Here's how the part is built. I have some questions about the finished solid (model axes, mm). Face numbers are marked on the shaded views. A direction names the side the tool comes from. Coordinates: 2 decimals unless noted, no trailing zeros. Write each loop counter-clockwise with the first axis right and the second up, starting at its lowest first coordinate (ties: lowest second). Pieces come first, ordered by that corner, then holes.
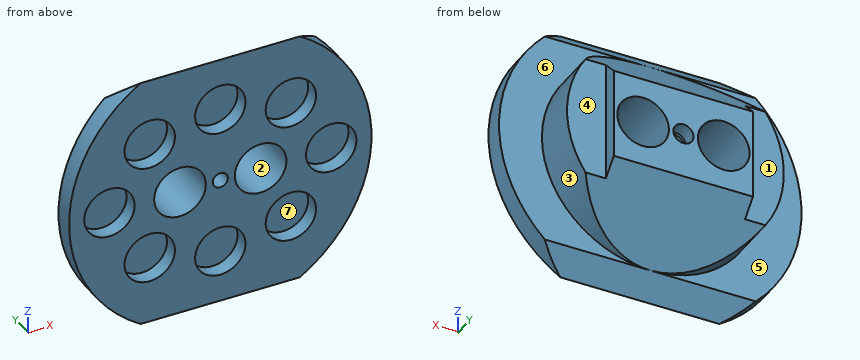
from build123d import *
from build123d.topology import SkipClean

# Parameters (mm, degrees)
SKETCH1_R                            = 30
BOSS_EXTRUDE1_DEPTH                  = 4
BOSS_EXTRUDE2_REACH                  = 44.615
BOSS_EXTRUDE2_END_RADIUS             = 30
BOSS_EXTRUDE2_DIRECTION_2_REACH      = 44.615
BOSS_EXTRUDE2_DIRECTION_2_END_RADIUS = 30
SKETCH3_OUTSIDE_W                    = 78.092
SKETCH3_OUTSIDE_H                    = 69.092
SKETCH3_OUTSIDE_R                    = 21.5
CUT_EXTRUDE2_DEPTH                   = 12.5
BOSS_EXTRUDE3_DEPTH                  = 18
BOSS_EXTRUDE4_DEPTH                  = 15
BOSS_EXTRUDE5_DEPTH                  = 15
CUT_EXTRUDE3_DEPTH                   = 44.292609069
CUT_EXTRUDE3_DEPTH_BACK              = 44.292609069
SKETCH8_R                            = 2
CUT_EXTRUDE8_DEPTH                   = 48.077064479
CUT_EXTRUDE8_DEPTH_BACK              = 48.077064479
CUT_EXTRUDE9_DEPTH                   = 59.659818207
CUT_EXTRUDE11_DEPTH                  = 20
CUT_EXTRUDE12_DEPTH                  = 20
CUT_EXTRUDE13_DEPTH                  = 20
CUT_EXTRUDE14_DEPTH                  = 44.292609069
CUT_EXTRUDE14_DEPTH_BACK             = 44.292609069
SKETCH25_W                           = 66.075437062
SKETCH25_H                           = 20.142243048
SKETCH26_R                           = 5.125
CUT_EXTRUDE15_DEPTH                  = 24
CUT_EXTRUDE17_DEPTH                  = 47.524187258
CUT_EXTRUDE17_DEPTH_BACK             = 47.524187258
SKETCH29_W                           = 7.7
SKETCH29_H                           = 3
CUT_EXTRUDE18_DEPTH                  = 47.524187258
CUT_EXTRUDE18_DEPTH_BACK             = 47.524187258
SKETCH31_W                           = 7.7
SKETCH31_H                           = 3
SKETCH34_R                           = 1.5
CUT_EXTRUDE21_DEPTH                  = 20
SKETCH35_R                           = 2
CUT_EXTRUDE22_DEPTH                  = 3
SKETCH37_R                           = 5
CUT_EXTRUDE23_DEPTH                  = 3


with BuildPart() as part:
    # Sketch1 → Boss-Extrude1 (new body)
    with BuildSketch(Plane(origin=(0, 0, 0), x_dir=(1, 0, 0), z_dir=(0, 1, 0))):
        with Locations(Location((0, 0, 0), (0, 0, 270))):
            Circle(SKETCH1_R)
    extrude(amount=BOSS_EXTRUDE1_DEPTH)

    # Boss-Extrude2: up to this cylinder (the profile starts inside it)
    with SkipClean():  # the faces are left unmerged after this step: merging them gives an invalid solid
        boss_extrude2_end = Plane(origin=(0, 9.396175, 0), z_dir=(0, -1, 0)) * Cylinder(BOSS_EXTRUDE2_END_RADIUS, 150.23, mode=Mode.PRIVATE)
        # Sketch2 → Boss-Extrude2 (add, up to the surface)
        with BuildSketch(Plane(origin=(0, 0, 0), x_dir=(0, 0, -1), z_dir=(1, 0, 0)), mode=Mode.PRIVATE) as boss_extrude2_sk1:
            Polygon((0, 4), (21.5, 4), (9, 16.5), (-9, 16.5), (-21.5, 4), align=None)
        boss_extrude2_tool1 = extrude(boss_extrude2_sk1.sketch, amount=BOSS_EXTRUDE2_REACH, mode=Mode.PRIVATE) & boss_extrude2_end
        add(boss_extrude2_tool1.solids().sort_by_distance((0, 9.396175, 0))[0])

    # Boss-Extrude2 direction 2: up to this cylinder (the profile starts inside it)
    with SkipClean():  # the faces are left unmerged after this step: merging them gives an invalid solid
        boss_extrude2_direction_2_end = Plane(origin=(0, 9.396175, 0), z_dir=(0, -1, 0)) * Cylinder(BOSS_EXTRUDE2_DIRECTION_2_END_RADIUS, 150.23, mode=Mode.PRIVATE)
        # Sketch2 → Boss-Extrude2 direction 2 (add, up to the surface)
        with BuildSketch(Plane(origin=(0, 0, 0), x_dir=(0, 0, -1), z_dir=(1, 0, 0)), mode=Mode.PRIVATE) as boss_extrude2_direction_2_sk1:
            Polygon((0, 4), (21.5, 4), (9, 16.5), (-9, 16.5), (-21.5, 4), align=None)
        boss_extrude2_direction_2_tool1 = extrude(boss_extrude2_direction_2_sk1.sketch, amount=-BOSS_EXTRUDE2_DIRECTION_2_REACH, mode=Mode.PRIVATE) & boss_extrude2_direction_2_end
        add(boss_extrude2_direction_2_tool1.solids().sort_by_distance((0, 9.396175, 0))[0])

    # SurfaceCut1
    split(bisect_by=Plane(origin=(0, 12.75, -12.75), x_dir=(1, 0, 0), z_dir=(0, 0.7071067811865558, -0.7071067811865392)), keep=Keep.BOTTOM)

    # SurfaceCut2
    split(bisect_by=Plane(origin=(0, 12.75, 12.75), x_dir=(1, 0, 0), z_dir=(0, 0.7071067811865509, 0.7071067811865442)), keep=Keep.BOTTOM)

    # Sketch3 outside → Cut-Extrude2 (cut)
    with BuildSketch(Plane(origin=(0, 4, 0), x_dir=(1, 0, 0), z_dir=(0, 1, 0))):
        Rectangle(SKETCH3_OUTSIDE_W, SKETCH3_OUTSIDE_H)
        Circle(SKETCH3_OUTSIDE_R, mode=Mode.SUBTRACT)
    extrude(amount=CUT_EXTRUDE2_DEPTH, mode=Mode.SUBTRACT)

    # Sketch5 → Boss-Extrude3 (add)
    with BuildSketch(Plane(origin=(0, 0, 0), x_dir=(-1, 0, 0), z_dir=(0, -1, 0))):
        Polygon((0, -6), (-17.5, -6), (-17.5, 6), (17.5, 6), (17.5, -6), align=None)
    extrude(amount=BOSS_EXTRUDE3_DEPTH)

    # Sketch6 → Boss-Extrude4 (add)
    with BuildSketch(Plane.XZ):
        Polygon((0, 15), (7, 15), (7, 6), (-7, 6), (-7, 15), align=None)
    extrude(amount=BOSS_EXTRUDE4_DEPTH)

    # Sketch7 → Boss-Extrude5 (add)
    with BuildSketch(Plane.XZ):
        Polygon((0, -15), (7, -15), (7, -6), (-7, -6), (-7, -15), align=None)
    extrude(amount=BOSS_EXTRUDE5_DEPTH)

    # Sketch8 → Cut-Extrude3 (cut, two sides: drawn at the far end of the back side and taken through both)
    with BuildSketch(Plane.XY.offset(-CUT_EXTRUDE3_DEPTH_BACK)):
        with Locations((-12.5, -12.5)):
            Circle(SKETCH8_R)
        with Locations((12.5, -12.5)):
            Circle(SKETCH8_R)
    extrude(amount=CUT_EXTRUDE3_DEPTH + CUT_EXTRUDE3_DEPTH_BACK, mode=Mode.SUBTRACT)

    # Sketch16 → Cut-Extrude8 (cut, two sides: drawn at the far end of the back side and taken through both)
    with BuildSketch(Plane.XY.offset(6).offset(-CUT_EXTRUDE8_DEPTH_BACK)):
        Polygon((17.5, -18), (17.5, -14.5), (14, -18), align=None)
        Polygon((-17.5, -18), (-14, -18), (-17.5, -14.5), align=None)
    extrude(amount=CUT_EXTRUDE8_DEPTH + CUT_EXTRUDE8_DEPTH_BACK, mode=Mode.SUBTRACT)

    # Sketch17 → Cut-Extrude9 (cut, through all)
    with BuildSketch(Plane(origin=(10.365975269, -9.674910251, -8.062425209), x_dir=(-0.3613483622370374, 0.337258471421235, -0.8693009171531012), z_dir=(0.6355070151731325, -0.5931398808282571, -0.49428323402354774))):
        Polygon((-2.372510104, -6.189601271), (7.980636686, -0.706686759), (7.980636686, -10.965829024), align=None)
    extrude(amount=CUT_EXTRUDE9_DEPTH, mode=Mode.SUBTRACT)

    # Sketch19 → Cut-Extrude11 (cut)
    with BuildSketch(Plane(origin=(-10.365975269, -9.674910251, -8.062425209), x_dir=(0.3613483622370374, 0.33725847142123494, -0.8693009171531012), z_dir=(0.6355070151731324, 0.5931398808282571, 0.4942832340235476))):
        Polygon((-2.372510104, -6.189601271), (7.980636686, -10.965829024), (7.980636686, -0.706686759), align=None)
    extrude(amount=-CUT_EXTRUDE11_DEPTH, mode=Mode.SUBTRACT)

    # Sketch20 → Cut-Extrude12 (cut)
    with BuildSketch(Plane(origin=(-10.365975269, -9.674910251, 8.062425209), x_dir=(-0.3613483622370374, -0.3372584714212349, -0.8693009171531013), z_dir=(0.6355070151731326, 0.593139880828257, -0.49428323402354757))):
        Polygon((2.372510104, -6.189601271), (-7.980636686, -0.706686759), (-7.980636686, -10.965829024), align=None)
    extrude(amount=-CUT_EXTRUDE12_DEPTH, mode=Mode.SUBTRACT)

    # Sketch21 → Cut-Extrude13 (cut)
    with BuildSketch(Plane(origin=(10.365975269, -9.674910251, 8.062425209), x_dir=(-0.3613483622370374, 0.3372584714212349, 0.8693009171531013), z_dir=(-0.6355070151731326, 0.593139880828257, -0.49428323402354757))):
        Polygon((-2.372510104, -6.189601271), (7.980636686, -0.706686759), (7.980636686, -10.965829024), align=None)
    extrude(amount=-CUT_EXTRUDE13_DEPTH, mode=Mode.SUBTRACT)

    # Sketch25 → Cut-Extrude14 (cut, two sides: drawn at the far end of the back side and taken through both)
    with BuildSketch(Plane.XY.offset(-CUT_EXTRUDE14_DEPTH_BACK)):
        with Locations((0, -10.071121524)):
            Rectangle(SKETCH25_W, SKETCH25_H)
    extrude(amount=CUT_EXTRUDE14_DEPTH + CUT_EXTRUDE14_DEPTH_BACK, mode=Mode.SUBTRACT)

    # Sketch26 → Cut-Extrude15 (cut)
    with BuildSketch(Plane(origin=(0, 16.5, 0), x_dir=(1, 0, 0), z_dir=(0, 1, 0))):
        with Locations(Location((-8, 0, 0), (0, 0, 270))):
            Circle(SKETCH26_R)
        with Locations(Location((8, 0, 0), (0, 0, 270))):
            Circle(SKETCH26_R)
    extrude(amount=-CUT_EXTRUDE15_DEPTH, mode=Mode.SUBTRACT)

    # Sketch29 → Cut-Extrude17 (cut, two sides: drawn at the far end of the back side and taken through both)
    with BuildSketch(Plane.XY.offset(6).offset(-CUT_EXTRUDE17_DEPTH_BACK)):
        with Locations((17.65, 15)):
            Rectangle(SKETCH29_W, SKETCH29_H)
    extrude(amount=CUT_EXTRUDE17_DEPTH + CUT_EXTRUDE17_DEPTH_BACK, mode=Mode.SUBTRACT)

    # Sketch31 → Cut-Extrude18 (cut, two sides: drawn at the far end of the back side and taken through both)
    with BuildSketch(Plane.XY.offset(6).offset(-CUT_EXTRUDE18_DEPTH_BACK)):
        with Locations((-17.65, 15)):
            Rectangle(SKETCH31_W, SKETCH31_H)
    extrude(amount=CUT_EXTRUDE18_DEPTH + CUT_EXTRUDE18_DEPTH_BACK, mode=Mode.SUBTRACT)

    # Sketch34 → Cut-Extrude21 (cut)
    with BuildSketch(Plane.XZ):
        with Locations(Location((0, 0, 0), (0, 0, 270))):
            Circle(SKETCH34_R)
    extrude(amount=-CUT_EXTRUDE21_DEPTH, mode=Mode.SUBTRACT)

    # Sketch35 → Cut-Extrude22 (cut)
    with BuildSketch(Plane(origin=(0, 16.5, 0), x_dir=(1, 0, 0), z_dir=(0, 1, 0))):
        with Locations(Location((0, 0, 0), (0, 0, 270))):
            Circle(SKETCH35_R)
    extrude(amount=-CUT_EXTRUDE22_DEPTH, mode=Mode.SUBTRACT)

    # Sketch37 → Cut-Extrude23 (cut)
    with BuildSketch(Plane.XZ):
        with Locations(Location((0, -15, 0), (0, 0, 270))):
            Circle(SKETCH37_R)
        with Locations(Location((0, 15, 0), (0, 0, 270))):
            Circle(SKETCH37_R)
        with Locations(Location((-22, 0, 0), (0, 0, 270))):
            Circle(SKETCH37_R)
        with Locations(Location((22, 0, 0), (0, 0, 270))):
            Circle(SKETCH37_R)
        with Locations(Location((-14, 12, 0), (0, 0, 270))):
            Circle(SKETCH37_R)
        with Locations(Location((14, 12, 0), (0, 0, 270))):
            Circle(SKETCH37_R)
        with Locations(Location((-14, -12, 0), (0, 0, 270))):
            Circle(SKETCH37_R)
        with Locations(Location((14, -12, 0), (0, 0, 270))):
            Circle(SKETCH37_R)
    extrude(amount=-CUT_EXTRUDE23_DEPTH, mode=Mode.SUBTRACT)


solid = part.part
1. Thinking about a two-plate mould opening in Z: for the marked faces 1, 2 and 3, which applies, pulls with the +Z half, pulls with the -Z half, needs draft (parallel to the pull), parting line crosses it, or undercut?
2. I want a section at B-B (x = 12). List the corners of the cut face in (y, z) for me.
3. I want a section at C-C (z = -3.5). List the corners of the cut face in (x, y) for me, then the cut area to 3 significant figures.
4. I want a section at D-D (z = -13.5). List the corners of the cut face in (x, y) for me.
5. If I drill on line 1 (X direction, y = 1.2, z = 0) (3 decimals); line 2 (X direction, y = 9.25, z = 0) (3 decimals); line 3 (X direction, y = 12.75, z = -4), over which ranges is the centre line in solid material (lowest first)?
6. On a 3-axis mill with a long thin cutter (end or side, diameter ignored), from which of +Z, -Z, +X, -X, +Y, -Y can I reach the whole of each face in a straight line? I mean the marked faces 4, 5, 6 and 7. Say none if no direction works.
7. I want a section at A-A (y = 14.75). List the corners of the cut face in (x, z) for me (3 decimals).
8. For pin 1 Ø5 at (x, z) = (21.5, 2) entering from -Y; pin 2 Ø16 at (x, z) = (0, 15) entering from -Y; pin 3 Ø1.5 at (y, z) = (15.5, 5.5) entering from +X; pin 4 Ø9 at (x, z) = (-20, 3) entering from +Y, each with a flat end and sliding along its axis, tell me the tip position at first contact or that it passes through.
Response values:
1. face 1: needs draft
1. face 2: undercut
1. face 3: parting line crosses it
2. outline: (0, -25.5) - (4, -21.5) - (4, -17.84) - (7.66, -17.84) - (16.5, -9) - (16.5, -3.2) - (0, -3.2) - (0, -7.42) - (3, -7.42) - (3, -16.58) - (0, -16.58) - close; (0, 3.2) - (16.5, 3.2) - (16.5, 9) - (7.66, 17.84) - (4, 17.84) - (4, 21.5) - (0, 25.5) - (0, 16.58) - (3, 16.58) - (3, 7.42) - (0, 7.42) - close
3. outline: (-29.8, 0) - (-25.57, 0) - (-25.57, 3) - (-18.43, 3) - (-18.43, 0) - (-11.74, 0) - (-11.74, 16.5) - (-13.8, 16.5) - (-13.8, 13.5) - (-21.21, 13.5) - (-21.21, 4) - (-29.8, 4) - close; (-4.26, 0) - (4.26, 0) - (4.26, 16.5) - (-4.26, 16.5) - close; (11.74, 0) - (18.43, 0) - (18.43, 3) - (25.57, 3) - (25.57, 0) - (29.8, 0) - (29.8, 4) - (21.21, 4) - (21.21, 13.5) - (13.8, 13.5) - (13.8, 16.5) - (11.74, 16.5) - close
3. area: 434 mm2
4. outline: (-26.79, 0) - (-18.77, 0) - (-18.77, 3) - (-9.23, 3) - (-9.23, 0) - (-4.77, 0) - (-4.77, 3) - (4.77, 3) - (4.77, 0) - (9.23, 0) - (9.23, 3) - (18.77, 3) - (18.77, 0) - (26.79, 0) - (26.79, 4) - (16.73, 4) - (16.73, 12) - (-16.73, 12) - (-16.73, 4) - (-26.79, 4) - close
5. line 1: x = -30 to -27, -17 to -13.125, -2.875 to -1.5, 1.5 to 2.875, 13.125 to 17, 27 to 30
5. line 2: x = -21.5 to -13.125, -2.875 to -1.5, 1.5 to 2.875, 13.125 to 21.5
5. line 3: x = -21.12 to -11.2, -4.8 to 4.8, 11.2 to 21.12
6. face 4: +Z, -Z, +X, +Y
6. face 5: -X, +Y
6. face 6: +X, +Y
6. face 7: -Y
7. outline: (-13.8, -10.75) - (13.8, -10.75) - (13.8, 10.75) - (-13.8, 10.75) - close; hole circle Ø10.25 at (-8, 0); hole circle Ø4 at (0, 0); hole circle Ø10.25 at (8, 0)
8. pin 1: stops at y = 3
8. pin 2: stops at y = 0
8. pin 3: stops at x = 13.8
8. pin 4: stops at y = 13.5
